```python
from build123d import *

# Parameters (mm, degrees)
BOSS_EXTRUDE1_DEPTH = 20
SKETCH2_R           = 20
CUT_EXTRUDE1_DEPTH  = 21
SKETCH3_W           = 16
SKETCH3_H           = 76
BOSS_EXTRUDE2_DEPTH = 150


with BuildPart() as part:
    # Sketch1 → Boss-Extrude1 (new body)
    with BuildSketch(Plane.XY):
        with BuildLine():
            Line((0, 80), (0, 0))
            Line((0, 0), (60, 0))
            ThreePointArc((60, 0), (88.284271247, 11.715728753), (100, 40))
            ThreePointArc((100, 40), (88.284271247, 68.284271247), (60, 80))
            Line((60, 80), (0, 80))
        make_face()
    extrude(amount=BOSS_EXTRUDE1_DEPTH)

    # Sketch2 → Cut-Extrude1 (cut, through all)
    with BuildSketch(Plane.XY.offset(20)):
        with Locations((60, 40)):
            Circle(SKETCH2_R)
    extrude(amount=-CUT_EXTRUDE1_DEPTH, mode=Mode.SUBTRACT)

    # Sketch3 → Boss-Extrude2 (add)
    with BuildSketch(Plane.ZY):
        with Locations((10, 40)):
            Rectangle(SKETCH3_W, SKETCH3_H)
    extrude(amount=BOSS_EXTRUDE2_DEPTH)


solid = part.part
```
Check sheet for the modelled part. Datum: model origin and axes. Units: mm. A direction names the side the tool comes from. Coordinates: 2 decimals unless noted, no trailing zeros. Order: outer loops, then holes, each group sorted by start corner. A loop starts at its lowest first (then second) coordinate and runs counter-clockwise, first axis right, second up. Notation, with made-up numbers: (32.25, 60) -> (81.25, 60) arc R12 cw to (81.25, 69) -> close; hole circle Ø5 at (-40, 5). An arc over 180 degrees is marked (long way). Write each question's results on one line, items separated by ' | '. Start each with the question number.
1) Material ranges on line 1 along Y through (x, z) = (60, 13); line 2 along Z through (x, y) = (-101, 67.5); line 3 along Y through (x, z) = (-135.5, 9), recorded low to high.
2) Section check A-A (y = 31.5). Enter the section's corners in (x, z), and give its area (3 significant figures).
3) Set-up check for faces 1 (the face through (38, 41, 20)), 2 (the face through (-74, 39, 2)), 3 (the face through (-74, 78, 10)), 4 (the face through (-74, 2, 10)), 5 (the face through (-74, 39, 18)): record each of +Z, -Z, +X, -X, +Y, -Y from which the full face is reachable in a straight line by a thin tool's end or side.
4) Draft check along X on faces 6 (the face through (-150, 41, 10)), 7 (the face through (30, 80, 10)), 8 (the face through (79.076, 46.007, 10.14)). Enter one of: pulls with the +X half, pulls with the -X half, needs draft (parallel to the pull), parting line crosses it, or undercut.
5) Section check B-B (z = 15.25). Enter the section's corners in (x, y), and give its area (3 significant figures).
6) Depth check by flat-ended pin: pin 1 (10 mm diameter, centred on y = 64.5, z = 10, fed in from +X); pin 2 (10 mm diameter, centred on x = -54.5, y = 17, fed in from +Z); pin 3 (6 mm diameter, centred on x = -122, y = 21.5, fed in from -Z). Enter the tip coordinate at first touch or a pass-through.
7) Section check C-C (y = 8). Enter the section's corners in (x, z), and give its area (3 significant figures).
8) Section check D-D (y = 52.5). Enter the section's corners in (x, z).
Checked values:
1) line 1: 0 to 20, 60 to 80 | line 2: 2 to 18 | line 3: 2 to 78
2) outline: (-150, 2) -> (0, 2) -> (0, 0) -> (41.9, 0) -> (41.9, 20) -> (0, 20) -> (0, 18) -> (-150, 18) -> close; (78.1, 0) -> (99.09, 0) -> (99.09, 20) -> (78.1, 20) -> close | area: 3,660 mm²
3) face 1: +Z, +X, -X, +Y, -Y | face 2: -Z, -X, +Y, -Y | face 3: +Z, -Z, -X, +Y | face 4: +Z, -Z, -X, -Y | face 5: +Z, -X, +Y, -Y
4) face 6: pulls with the -X half | face 7: needs draft | face 8: undercut
5) outline: (-150, 2) -> (0, 2) -> (0, 0) -> (60, 0) arc R40 ccw to (60, 80) -> (0, 80) -> (0, 78) -> (-150, 78) -> close; hole circle Ø40 at (60, 40) | area: 17,500 mm²
6) pin 1: x = 94.92 | pin 2: z = 18 | pin 3: z = 2
7) outline: (-150, 2) -> (0, 2) -> (0, 0) -> (84, 0) -> (84, 20) -> (0, 20) -> (0, 18) -> (-150, 18) -> close | area: 4,080 mm²
8) outline: (-150, 2) -> (0, 2) -> (0, 0) -> (44.39, 0) -> (44.39, 20) -> (0, 20) -> (0, 18) -> (-150, 18) -> close; (75.61, 0) -> (98, 0) -> (98, 20) -> (75.61, 20) -> close
